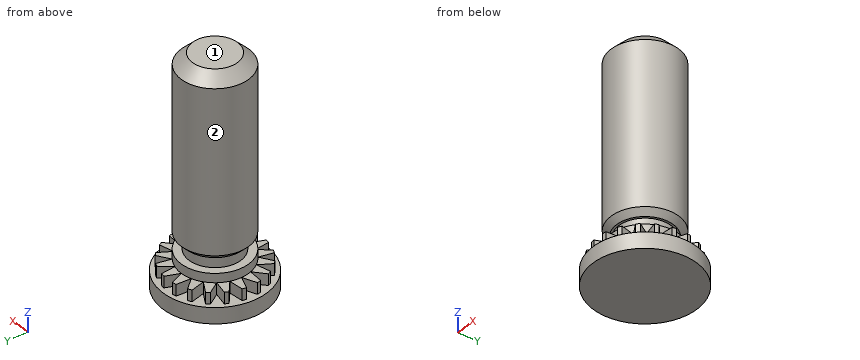
```python
from build123d import *

# Parameters (mm, degrees)
SKETCH_1_R               = 2.3
EXTRUDE_1_DEPTH          = 1.2
SKETCH_2_R               = 1.5
EXTRUDE_2_DEPTH          = 1.5
CUT_EXTRUDE_1_DEPTH      = 0.5
PATTERN_CIRCULAR_1_COUNT = 20
SKETCH_4_W               = 0.35
SKETCH_4_H               = 0.5
SKETCH_6_W               = 7.3
SKETCH_6_H               = 1.5
CHAMFER_2_SIZE           = 0.5
CUT_EXTRUDE_START        = -0.5
SKETCH_7_R               = 2.3
SKETCH_7_R_2             = 2.1
CUT_EXTRUDE_2_DEPTH      = 0.5


with BuildPart() as part:
    # Эскиз1 → Вытянуть1 (new body)
    with BuildSketch(Plane.XY):
        Circle(SKETCH_1_R)
    extrude(amount=EXTRUDE_1_DEPTH)

    # Эскиз2 → Вытянуть2 (add)
    with BuildSketch(Plane.XY.offset(1.2)):
        Circle(SKETCH_2_R)
    extrude(amount=EXTRUDE_2_DEPTH)

    # Эскиз3 → Вырез-Вытянуть1 (cut)
    with BuildSketch(Plane.XY.offset(1.2)):
        Polygon((-0.33137085, 2.3), (0.33137085, 2.3), (0, 1.5), align=None)
    cut_extrude_1 = extrude(amount=-CUT_EXTRUDE_1_DEPTH, mode=Mode.SUBTRACT)

    # Круговой массив1: Вырез-Вытянуть1 ×20 about axis
    pattern_circular_1_axis = Axis((0, 0, 0), (0, 0, 1))
    for i in range(1, PATTERN_CIRCULAR_1_COUNT):
        add(cut_extrude_1.rotate(pattern_circular_1_axis, i * 360 / PATTERN_CIRCULAR_1_COUNT), mode=Mode.SUBTRACT)

    # Эскиз4 → Вырез-Повернуть1 (revolve, cut)
    with BuildSketch(Plane(origin=(0, 0, 0), x_dir=(1, 0, 0), z_dir=(0, 1, 0))):
        with Locations((1.325, -1.85)):
            Rectangle(SKETCH_4_W, SKETCH_4_H)
    revolve(axis=Axis((0, 0, 10.642619983), (0, 0, -1)), mode=Mode.SUBTRACT)

    # Эскиз6 → Повернуть1 (revolve)
    with BuildSketch(Plane(origin=(0, 0, 0), x_dir=(0, 0, -1), z_dir=(1, 0, 0)), mode=Mode.PRIVATE) as revolve_1_sk:
        with Locations((-6.35, -0.75)):
            Rectangle(SKETCH_6_W, SKETCH_6_H)
    revolve(revolve_1_sk.sketch.rotate(Axis((0, 0, 2.7), (0, 0, 1)), 278.047567557), axis=Axis((0, 0, 2.7), (0, 0, 1)))

    # Фаска2
    # the kernel refuses this chamfer: 0.5 mm, written as the material it takes off along each edge
    with BuildSketch(Plane(origin=(0, 0, 10), x_dir=(-0.9901521845161062, -0.1399951838385265, 0), z_dir=(-0.1399951838385265, 0.9901521845161062, 0))) as chamfer_2_piece_1:
        Polygon((1.5, -CHAMFER_2_SIZE), (1.5 - CHAMFER_2_SIZE, 0), (1.5, 0), align=None)
    revolve(axis=Axis((0, 0, 10), (0, 0, 1)), mode=Mode.SUBTRACT)

    # Эскиз7 → Вырез-Вытянуть2 (cut)
    with BuildSketch(Plane.XY.offset(1.2).offset(CUT_EXTRUDE_START)):
        with Locations(Location((0, 0, 0), (0, 0, 180))):
            Circle(SKETCH_7_R)
        Circle(SKETCH_7_R_2, mode=Mode.SUBTRACT)
    extrude(amount=CUT_EXTRUDE_2_DEPTH, mode=Mode.SUBTRACT)

    # Фаска3
    # the kernel refuses this chamfer: 0.25 mm, written as the material it takes off along each edge
    with BuildSketch(Plane(origin=(0, 0, 2.1), x_dir=(1, 0, 0), z_dir=(0, 1, 0))) as chamfer_3_piece_1:
        with BuildLine():
            Line((1.242928932, 0.007071068), (1.507071068, -0.257071068))
            Line((1.507071068, -0.257071068), (1.512071068, -0.257071068))
            ThreePointArc((1.512071068, -0.257071068), (1.505, -0.128535534), (1.505, 0))
            Line((1.505, 0), (1.5, 0.005))
            ThreePointArc((1.5, 0.005), (1.371464466, 0.005), (1.242928932, 0.012071068))
            Line((1.242928932, 0.012071068), (1.242928932, 0.007071068))
        make_face()
    revolve(axis=Axis((0, 0, 2.1), (0, 0, -1)), mode=Mode.SUBTRACT)


solid = part.part
```
Source: CAD feature listing. Evaluate the final solid. Frame: model axes, mm. Face numbers are marked on the shaded views. A direction names the side the tool comes from. Round coordinates to 2 decimals unless told otherwise and drop trailing zeros. Write each loop counter-clockwise with the first axis right and the second up, starting at its lowest first coordinate (ties: lowest second). Pieces come first, ordered by that corner, then holes. Notation, with made-up numbers: M -31,-24 L 8,-24 A16 ccw 8,-6 Z; hole C 51.25,4 d6. An arc over 180 degrees is marked long. Answer as a JSON object with one key per item and string values. Group by question number.
(1) Reachability of the marked faces 1 and 2 from +Z, -Z, +X, -X, +Y, -Y: full face, straight path, thin tool, end or side. Return the list, or none.
(2) First-contact query: pin 1 (0.5 mm diameter, centred on x = -1, y = 1, fed in from +Z); pin 2 (1 mm diameter, centred on y = 0.5, z = 7, fed in from -X); pin 3 (0.5 mm diameter, centred on x = -1.5, y = 0, fed in from +Z). Flat tips, straight axial feed; report the tip coordinate or a pass-through.
(3) Ray query, line 1 (Z direction, x = 0.2, y = 1.6); line 2 (Z direction, x = -1.85, y = -0.7); line 3 (Y direction, x = -1.15, z = 1.25). Return the intervals inside material, ascending. Write a range as [from, to].
(4) Section query A-A on z = 7.5. Output: boundary loops of the cut face in (x, y), then the cut area to 3 significant figures.
Computed values:
{
 "1": {"face 1": "+Z, +X, -X, +Y, -Y", "face 2": "+Z"},
 "2": {"pin 1": "z = 9.84", "pin 2": "x = -1.5", "pin 3": "z = 9.75"},
 "3": {"line 1": "[0, 1.2]", "line 2": "[0, 0.7]", "line 3": "[-0.96, 0.96]"},
 "4": {"outline": "C 0,0 d3", "area": "7.07 mm^2"}
}
